Verification items for the finished model (mm, model axes). A direction names the side the tool comes from. Coordinates: 2 decimals unless noted, no trailing zeros. Order: outer loops, then holes, each group sorted by start corner. A loop starts at its lowest first (then second) coordinate and runs counter-clockwise, first axis right, second up. Notation, with made-up numbers: M 55.5,-6.75 L 109.5,-6.75 A24 ccw 109.5,10.25 Z; hole C 52,78.5 d1. An arc over 180 degrees is marked long. Return JSON: item names as keys, results as strings.
```python
from build123d import *

# Parameters (mm, degrees)
SKETCH1_W           = 15
SKETCH1_H           = 200
BOSS_EXTRUDE1_DEPTH = 10
CUT_EXTRUDE1_DEPTH  = 210
SKETCH3_W           = 5
SKETCH3_H           = 8
BOSS_EXTRUDE2_DEPTH = 20
CUT_EXTRUDE3_DEPTH  = 40
SKETCH6_W           = 5
SKETCH6_H           = 15
CUT_EXTRUDE4_DEPTH  = 40
SKETCH7_R           = 1.6
CUT_EXTRUDE5_DEPTH  = 24
CHAMFER1_SIZE       = 2
CHAMFER2_SIZE       = 2
CHAMFER3_SIZE       = 2
CHAMFER4_SIZE       = 2
FILLET1_R           = 2


with BuildPart() as part:
    # Sketch1 → Boss-Extrude1 (new body)
    with BuildSketch(Plane(origin=(0, 0, 0), x_dir=(1, 0, 0), z_dir=(0, 1, 0))):
        Rectangle(SKETCH1_W, SKETCH1_H)
    extrude(amount=BOSS_EXTRUDE1_DEPTH)

    # Sketch2 → Cut-Extrude1 (cut)
    with BuildSketch(Plane.XY.offset(100)):
        Polygon((-2.5, 10), (-4.5, 5), (4.5, 5), (2.5, 10), align=None)
    extrude(amount=-CUT_EXTRUDE1_DEPTH, mode=Mode.SUBTRACT)

    # Sketch3 → Boss-Extrude2 (add)
    with BuildSketch(Plane.XZ):
        with Locations((-10, -96)):
            Rectangle(SKETCH3_W, SKETCH3_H)
        with Locations((10, -96)):
            Rectangle(SKETCH3_W, SKETCH3_H)
    extrude(amount=-BOSS_EXTRUDE2_DEPTH)

    # Sketch4 → Cut-Extrude3 (cut)
    with BuildSketch(Plane(origin=(12.5, 0, 0), x_dir=(0, 0, -1), z_dir=(1, 0, 0))):
        Polygon((96.5, 17.5), (98, 17.5), (98, 15.5), (100, 15.5), (100, 13.5), (98, 13.5), (98, 11.5), (96.5, 11.5), align=None)
    extrude(amount=-CUT_EXTRUDE3_DEPTH, mode=Mode.SUBTRACT)

    # Sketch6 → Cut-Extrude4 (cut)
    with BuildSketch(Plane(origin=(0, 5, 0), x_dir=(1, 0, 0), z_dir=(0, 1, 0))):
        with Locations((0, -77.5)):
            Rectangle(SKETCH6_W, SKETCH6_H)
    extrude(amount=-CUT_EXTRUDE4_DEPTH, mode=Mode.SUBTRACT)

    # Sketch7 → Cut-Extrude5 (cut)
    with BuildSketch(Plane(origin=(7.5, 0, 0), x_dir=(0, 0, -1), z_dir=(1, 0, 0))):
        with Locations((-73.75, 2.5)):
            Circle(SKETCH7_R)
    extrude(amount=-CUT_EXTRUDE5_DEPTH, mode=Mode.SUBTRACT)

    # Chamfer1
    # the kernel refuses this chamfer: 2 mm, written as the material it adds along each edge
    with BuildSketch(Plane(origin=(-7.5, 10, -100), x_dir=(0.9996219169112968, -0.027495876610586487, 0), z_dir=(0, 0, 1))) as chamfer1_piece_1_section:
        Polygon((CHAMFER1_SIZE * 0.999621916911, CHAMFER1_SIZE * 0.0274958766106), (-CHAMFER1_SIZE * 0.0274958766106, CHAMFER1_SIZE * 0.999621916911), (0, 0), align=None)
    chamfer1_piece_1 = extrude(amount=8, mode=Mode.PRIVATE)
    chamfer1_piece_1 = split(chamfer1_piece_1, bisect_by=Plane(origin=(-6.8, 11.5, -99), z_dir=(0, -1, 0)), keep=Keep.TOP, mode=Mode.PRIVATE)
    add(chamfer1_piece_1)
    with BuildSketch(Plane(origin=(-7.5, 10, -100), x_dir=(0.9996219169112968, -0.027495876610586487, 0), z_dir=(0, 0, 1))) as chamfer1_piece_2_section:
        Polygon((CHAMFER1_SIZE * 0.999621916911, CHAMFER1_SIZE * 0.0274958766106), (-CHAMFER1_SIZE * 0.0274958766106, CHAMFER1_SIZE * 0.999621916911), (0, 0), align=None)
    chamfer1_piece_2 = extrude(amount=13.143365976, mode=Mode.PRIVATE)
    chamfer1_piece_2 = split(chamfer1_piece_2, bisect_by=Plane(origin=(-7.333333333, 11.666666667, -98), z_dir=(0, 0, -1)), keep=Keep.TOP, mode=Mode.PRIVATE)
    add(chamfer1_piece_2)
    with BuildSketch(Plane(origin=(-7.5, 10, -105.143365976), x_dir=(0.9996219169112968, -0.027495876610586487, 0), z_dir=(0, 0, 1))) as chamfer1_piece_3_section:
        Polygon((CHAMFER1_SIZE * 0.999621916911, CHAMFER1_SIZE * 0.0274958766106), (-CHAMFER1_SIZE * 0.0274958766106, CHAMFER1_SIZE * 0.999621916911), (0, 0), align=None)
    chamfer1_piece_3 = extrude(amount=13.143365976, mode=Mode.PRIVATE)
    chamfer1_piece_3 = split(chamfer1_piece_3, bisect_by=Plane(origin=(-7.333333333, 11.666666667, -96.5), z_dir=(0, 0, 1)), keep=Keep.TOP, mode=Mode.PRIVATE)
    add(chamfer1_piece_3)
    with BuildSketch(Plane(origin=(7.5, 10, -92), x_dir=(-0.9996219169112968, -0.027495876610586487, 0), z_dir=(0, 0, -1))) as chamfer1_piece_4_section:
        Polygon((CHAMFER1_SIZE * 0.999621916911, CHAMFER1_SIZE * 0.0274958766106), (-CHAMFER1_SIZE * 0.0274958766106, CHAMFER1_SIZE * 0.999621916911), (0, 0), align=None)
    chamfer1_piece_4 = extrude(amount=8, mode=Mode.PRIVATE)
    chamfer1_piece_4 = split(chamfer1_piece_4, bisect_by=Plane(origin=(6.8, 11.5, -94.25), z_dir=(0, -1, 0)), keep=Keep.TOP, mode=Mode.PRIVATE)
    add(chamfer1_piece_4)
    with BuildSketch(Plane(origin=(7.5, 10, -92), x_dir=(-0.9996219169112968, -0.027495876610586487, 0), z_dir=(0, 0, -1))) as chamfer1_piece_5_section:
        Polygon((CHAMFER1_SIZE * 0.999621916911, CHAMFER1_SIZE * 0.0274958766106), (-CHAMFER1_SIZE * 0.0274958766106, CHAMFER1_SIZE * 0.999621916911), (0, 0), align=None)
    chamfer1_piece_5 = extrude(amount=13.143365976, mode=Mode.PRIVATE)
    chamfer1_piece_5 = split(chamfer1_piece_5, bisect_by=Plane(origin=(7.333333333, 11.666666667, -96.5), z_dir=(0, 0, 1)), keep=Keep.TOP, mode=Mode.PRIVATE)
    add(chamfer1_piece_5)
    with BuildSketch(Plane(origin=(7.5, 10, -86.856634024), x_dir=(-0.9996219169112968, -0.027495876610586487, 0), z_dir=(0, 0, -1))) as chamfer1_piece_6_section:
        Polygon((CHAMFER1_SIZE * 0.999621916911, CHAMFER1_SIZE * 0.0274958766106), (-CHAMFER1_SIZE * 0.0274958766106, CHAMFER1_SIZE * 0.999621916911), (0, 0), align=None)
    chamfer1_piece_6 = extrude(amount=13.143365976, mode=Mode.PRIVATE)
    chamfer1_piece_6 = split(chamfer1_piece_6, bisect_by=Plane(origin=(7.333333333, 11.666666667, -98), z_dir=(0, 0, -1)), keep=Keep.TOP, mode=Mode.PRIVATE)
    add(chamfer1_piece_6)

    # Chamfer2
    chamfer2_edges = [part.edges().sort_by_distance(p)[0] for p in [
        (7.5, 10, 4),
        (-7.5, 10, 4),
    ]]
    chamfer(chamfer2_edges, length=CHAMFER2_SIZE)

    # Chamfer3
    chamfer3_edges = [part.edges().sort_by_distance(p)[0] for p in [
        (7.5, 4, -92),
        (-7.5, 4, -92),
    ]]
    chamfer(chamfer3_edges, length=CHAMFER3_SIZE)

    # Chamfer4
    chamfer4_edges = [part.edges().sort_by_distance(p)[0] for p in [
        (-10, 20, -92),
        (10, 20, -92),
    ]]
    chamfer(chamfer4_edges, length=CHAMFER4_SIZE)

    # Fillet1
    fillet1_edges = [part.edges().sort_by_distance(p)[0] for p in [
        (12.5, 9, -92),
        (-12.5, 9, -92),
    ]]
    fillet(fillet1_edges, radius=FILLET1_R)


solid = part.part
```
Q1. Cross-section at A-A, the plane z = 83. Record the boundary of the cut face in (x, y), and give its area (3 significant figures).
Values:
{"outline": "M -7.5,0 L -2.5,0 L -2.5,5 L -4.5,5 L -2.5,10 L -5.5,10 L -7.5,8 Z; M 2.5,0 L 7.5,0 L 7.5,8 L 5.5,10 L 2.5,10 L 4.5,5 L 2.5,5 Z", "area": "86.0 mm^2"}
Q2. Cross-section at B-B, the plane z = -13.5. Record the boundary of the cut face in (x, y), and give its area (3 significant figures).
Values:
{"outline": "M -7.5,0 L 7.5,0 L 7.5,8 L 5.5,10 L 2.5,10 L 4.5,5 L -4.5,5 L -2.5,10 L -5.5,10 L -7.5,8 Z", "area": "111 mm^2"}
Q3. Tool access check on faces 5 (the face through (2.5, 3, 78)), 6 (the face through (7.5, 16, -95)), 7 (the face through (-6.6, 8.9, 5.3)), 8 (the face through (-3.5, 7.5, 1.4)), 9 (the face through (-7.5, 4, 6)). Record the directions out of +Z, -Z, +X, -X, +Y, -Y that give a thin tool (end or side, any length) a straight path to the whole face; none if there is none.
Values:
{"face 5": "+Y, -Y", "face 6": "+Z, -Z, +Y", "face 7": "+Z, -X, +Y", "face 8": "+Z, -Z", "face 9": "+Z, -X, +Y, -Y"}
Q4. Go/stop test with flat-tipped pins: pin 1 (7 mm diameter, centred on x = -0.5, z = -44.5, fed in from +Y); pin 2 (4 mm diameter, centred on y = 6, z = -13, fed in from -X); pin 3 (1.9 mm diameter, centred on y = 2.5, z = 73.75, fed in from +X); pin 4 (5.5 mm diameter, centred on y = 2, z = 77, fed in from +X). Record where each tip stops, or that it passes through.
Values:
{"pin 1": "y = 10", "pin 2": "x = -7.5", "pin 3": "through", "pin 4": "x = 7.5"}
Q5. Material ranges on line 1 along Z through (x, y) = (0.5, 1); line 2 along Y through (x, z) = (-5.35, 73.75); line 3 along X through (y, z) = (2, 70.5), recorded low to high.
Values:
{"line 1": "-100 to 70, 85 to 100", "line 2": "0 to 0.9, 4.1 to 10", "line 3": "-7.5 to -2.5, 2.5 to 7.5"}
Q6. Draft check along Z on faces 1 (the face through (0, 4, -100)), 2 (the face through (-10, 15, -96.5)), 3 (the face through (9, 11, -92)), 4 (the face through (-4.965, 2.981, 72.224)). Enter one of: pulls with the +Z half, pulls with the -Z half, needs draft (parallel to the pull), parting line crosses it, or undercut.
Values:
{"face 1": "pulls with the -Z half", "face 2": "undercut", "face 3": "pulls with the +Z half", "face 4": "undercut"}
